The model under review builds one solid part; all positions refer to its coordinate system, in mm. Face numbers are marked on the shaded views. Coordinates: 2 decimals unless noted, no trailing zeros. Order: outer loops, then holes, each group sorted by start corner. A loop starts at its lowest first (then second) coordinate and runs counter-clockwise, first axis right, second up.
from build123d import *

# Parameters (mm, degrees)
F0_W     = 44
F0_H     = 44
F0_R     = 3.5
F0_R_2   = 1.75
F0_R_3   = 19
F0_W_2   = 8.5
F0_H_2   = 16
F1_DEPTH = 3
F2_DEPTH = 10
F3_R     = 1.75
F4_R     = 2


with BuildPart() as f1:
    # F0 (on Top) → F1 (new body)
    with BuildSketch(Plane.XY):
        Rectangle(F0_W, F0_H)
        with Locations((-16, -16)):
            Circle(F0_R, mode=Mode.SUBTRACT)
        with Locations((16, -16)):
            Circle(F0_R, mode=Mode.SUBTRACT)
        with Locations((-16, 16)):
            Circle(F0_R_2, mode=Mode.SUBTRACT)
        Circle(F0_R_3, mode=Mode.SUBTRACT)
        with Locations((16, 16)):
            Circle(F0_R, mode=Mode.SUBTRACT)
        Polygon((-22, -22), (-22, 22), (-42, 22), (-46, 22), (-46, -22), align=None)
        with Locations((-30.25, -10)):
            Rectangle(F0_W_2, F0_H_2, mode=Mode.SUBTRACT)
        with BuildLine():
            ThreePointArc((-42, 16.25), (-40.25, 18), (-38.5, 16.25))
            Line((-38.5, 16.25), (-38.5, -16.25))
            ThreePointArc((-38.5, -16.25), (-40.25, -18), (-42, -16.25))
            Line((-42, -16.25), (-42, 16.25))
        make_face(mode=Mode.SUBTRACT)
        with Locations((-30.25, 10)):
            Rectangle(F0_W_2, F0_H_2, mode=Mode.SUBTRACT)
    extrude(amount=F1_DEPTH)

    # F0 (on Top) → F2 (join)
    with BuildSketch(Plane.XY):
        with Locations((16, 16)):
            Circle(F0_R)
        with Locations((16, 16)):
            Circle(F0_R_2, mode=Mode.SUBTRACT)
        with Locations((16, -16)):
            Circle(F0_R)
        with Locations((16, -16)):
            Circle(F0_R_2, mode=Mode.SUBTRACT)
        with Locations((-16, -16)):
            Circle(F0_R)
        with Locations((-16, -16)):
            Circle(F0_R_2, mode=Mode.SUBTRACT)
    extrude(amount=F2_DEPTH)

    # F3
    f3_edges = [f1.edges().sort_by_distance(p)[0] for p in [
        (-34.5, 18, 1.5),
        (-26, 18, 1.5),
        (-34.5, 2, 1.5),
        (-26, 2, 1.5),
        (-34.5, -18, 1.5),
        (-26, -18, 1.5),
        (-34.5, -2, 1.5),
        (-26, -2, 1.5),
    ]]
    fillet(f3_edges, radius=F3_R)

    # F4
    f4_edges = [f1.edges().sort_by_distance(p)[0] for p in [
        (-46, 22, 1.5),
        (-46, -22, 1.5),
        (22, -22, 1.5),
        (22, 22, 1.5),
    ]]
    fillet(f4_edges, radius=F4_R)


solid = f1.part
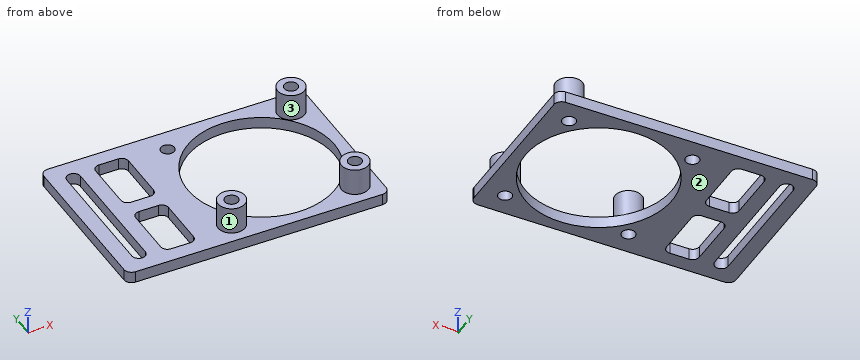
(1) The part is to be moulded in two halves that separate along Y. For the marked faces 1, 2 and 3, say which applies: +Y half, -Y half, draft (parallel to the pull), parting line (faces both ways), or undercut.
(2) Insertion check: pin 1 Ø4 at (x, y) = (-36.5, -16.5) entering from +Z; pin 2 Ø3 at (x, z) = (11.5, 6) entering from +Y; pin 3 Ø6 at (y, z) = (-12.5, 7.5) entering from -X. Each pin has a flat end and moves straight along its axis. Give the tip position at first contact, or say it passes through.
(3) Consider section C-C (z = 6.75). Give the boundary of the cut face in (x, y), then the cut area to 3 significant figures.
(4) Consider section B-B (x = 0). Give the boundary of the cut face in (y, z), then the cut area to 3 significant figures.
(5) Consider section D-D (x = -31.5). Give the boundary of the cut face in (y, z), then the cut area to 3 significant figures.
(6) Wall thickness on line 1 (Y direction, x = -16, z = 3.25); line 2 (Y direction, x = -31.5, z = 1.25); line 3 (Z direction, x = -40.5, y = 18.5): over which ranges is each line inside the solid? List them lowest first.
(7) Consider section A-A (y = 0). Give the boundary of the cut face in (x, z).
Findings:
1. face 1: parting line
1. face 2: draft
1. face 3: undercut
2. pin 1: stops at z = 3
2. pin 2: stops at y = 17.8
2. pin 3: stops at x = -19.46
3. outline: circle Ø7 at (-16, -16); circle Ø7 at (16, -16); circle Ø7 at (16, 16); hole circle Ø3.5 at (-16, -16); hole circle Ø3.5 at (16, -16); hole circle Ø3.5 at (16, 16)
3. area: 86.6 mm2
4. outline: (-22, 0) - (-19, 0) - (-19, 3) - (-22, 3) - close; (19, 0) - (22, 0) - (22, 3) - (19, 3) - close
4. area: 18.0 mm2
5. outline: (-22, 0) - (-18, 0) - (-18, 3) - (-22, 3) - close; (-2, 0) - (2, 0) - (2, 3) - (-2, 3) - close; (18, 0) - (22, 0) - (22, 3) - (18, 3) - close
5. area: 36.0 mm2
6. line 1: y = -19.5 to -17.75, -14.25 to -12.5
6. line 2: y = -22 to -18, -2 to 2, 18 to 22
6. line 3: z = 0 to 3
7. outline: (-46, 0) - (-42, 0) - (-42, 3) - (-46, 3) - close; (-38.5, 0) - (-19, 0) - (-19, 3) - (-38.5, 3) - close; (19, 0) - (22, 0) - (22, 3) - (19, 3) - close
